Model file for the job. Use its own axes, mm. Face numbers are marked on the shaded views. A direction names the side the tool comes from. Give positions to 0.01 mm unless a question says otherwise; leave off trailing zeros. Loops run counter-clockwise (first coordinate to the right, second up) from the corner with the lowest first, then second, coordinate; pieces in that order, holes last. Notation, with made-up numbers: (-21, -2.5) - (29, -2.5) arc R29 cw to (29, 20.5) - close; hole circle Ø2 at (42, 1). An arc over 180 degrees is marked (long way). Use a Markdown table: item, result.
from build123d import *

# Parameters (mm, degrees)
EXTRUDE_1_DEPTH     = 60
SKETCH_3_W          = 10
SKETCH_3_H          = 40
CUT_EXTRUDE_2_DEPTH = 148.102218349
EXTRUDE_4_DEPTH     = 30
EXTRUDE_5_DEPTH     = 30
SKETCH_9_R          = 5
EXTRUDE_6_DEPTH     = 30
SKETCH_10_R         = 2.5
EXTRUDE_7_DEPTH     = 10
SKETCH_11_W         = 20.162650783
SKETCH_11_H         = 30
CUT_EXTRUDE_3_DEPTH = 10


with BuildPart() as part:
    # 草图1 → 凸台-拉伸1 (new body)
    with BuildSketch(Plane(origin=(0, 0, 0), x_dir=(1, 0, 0), z_dir=(0, 1, 0))):
        Polygon((0, 0), (120.162650783, 0), (120.162650783, 60), (100, 60), (100, 20), (0, 20), align=None)
    extrude(amount=EXTRUDE_1_DEPTH)

    # 草图3 → 切除-拉伸2 (cut, through all)
    with BuildSketch(Plane(origin=(120.162650783, 0, 0), x_dir=(0, 0, -1), z_dir=(1, 0, 0))):
        with Locations((55, 30)):
            Rectangle(SKETCH_3_W, SKETCH_3_H)
    extrude(amount=-CUT_EXTRUDE_2_DEPTH, mode=Mode.SUBTRACT)

    # 草图7 → 凸台-拉伸4 (add)
    with BuildSketch(Plane(origin=(0, 60, 0), x_dir=(1, 0, 0), z_dir=(0, 1, 0))):
        Polygon((0, 20), (0, 0), (120.162650783, 0), (120.162650783, 60), (100, 60), (100, 20), align=None)
    extrude(amount=EXTRUDE_4_DEPTH)

    # 草图8 → 凸台-拉伸5 (add)
    with BuildSketch(Plane.XZ):
        Polygon((0, -20), (0, 0), (120.162650783, 0), (120.162650783, -60), (100, -60), (100, -20), align=None)
    extrude(amount=EXTRUDE_5_DEPTH)

    # 草图9 → 凸台-拉伸6 (add)
    with BuildSketch(Plane(origin=(0, 0, -20), x_dir=(-1, 0, 0), z_dir=(0, 0, -1))):
        with Locations(Location((-10, -20, 0), (0, 0, 180))):
            Circle(SKETCH_9_R)
        with Locations(Location((-10, 80, 0), (0, 0, 180))):
            Circle(SKETCH_9_R)
    extrude(amount=EXTRUDE_6_DEPTH)

    # 草图10 → 凸台-拉伸7 (add)
    with BuildSketch(Plane(origin=(0, 0, -50), x_dir=(-1, 0, 0), z_dir=(0, 0, -1))):
        with Locations((-10, -20)):
            Circle(SKETCH_10_R)
        with Locations((-10, 80)):
            Circle(SKETCH_10_R)
    extrude(amount=EXTRUDE_7_DEPTH)

    # 草图11 → 切除-拉伸3 (cut)
    with BuildSketch(Plane(origin=(0, 0, -60), x_dir=(-1, 0, 0), z_dir=(0, 0, -1))):
        with Locations((-110.081325392, -5)):
            Rectangle(SKETCH_11_W, SKETCH_11_H)
        with Locations((-110.081325392, 65)):
            Rectangle(SKETCH_11_W, SKETCH_11_H)
    extrude(amount=-CUT_EXTRUDE_3_DEPTH, mode=Mode.SUBTRACT)


solid = part.part
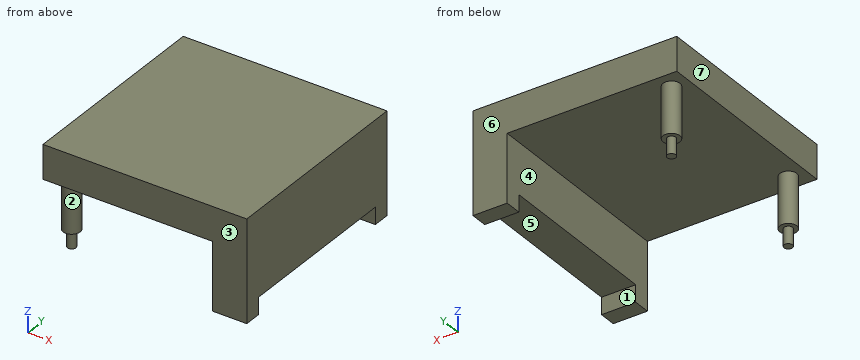
(1) Slice it at D-D, the plane x = 10. Write the cut outline in (y, z), plus the area to 3 significant figures.
Computed:
| item | result |
|---|---|
| outline | (-30, -20) - (-25, -20) - (-25, -50) - (-22.5, -50) - (-22.5, -60) - (-17.5, -60) - (-17.5, -50) - (-15, -50) - (-15, -20) - (75, -20) - (75, -50) - (77.5, -50) - (77.5, -60) - (82.5, -60) - (82.5, -50) - (85, -50) - (85, -20) - (90, -20) - (90, 0) - (-30, 0) - close |
| area | 3,100 mm² |
(2) Pin check, flat tips, straight feed: P1, Ø6, axis at x = 57, y = 3.5, coming from the -Z side; P2, Ø2, axis at y = 68.5, z = -40, coming from the -X side; P3, Ø6, axis at x = 113.5, y = 19, coming from the -Z side; P4, Ø1.5, axis at x = 102.5, y = -3.5, coming from the +Z side. Stop position of each tip, or through.
Computed:
| item | result |
|---|---|
| P1 | z = -20 |
| P2 | x = 100 |
| P3 | z = -50 |
| P4 | z = 0 |
(3) Drill centre lines: probe 1 along Z at (x, y) = (69.5, 65); probe 2 along X at (y, z) = (9, -34); probe 3 along Z at (x, y) = (101, 2.5). Where is each one in solid material? Low to high. Write a range as [from, to].
Computed:
| item | result |
|---|---|
| probe 1 | [-20, 0] |
| probe 2 | [100, 120.16] |
| probe 3 | [-50, 0] |
(4) 3-axis set-ups, long thin cutter, end or side, ignore diameter. For the marked faces 1, 2, 3 and 4: which of +Z, -Z, +X, -X, +Y, -Y reach the whole face in a straight line?
Computed:
| item | result |
|---|---|
| face 1 | -Z, +X |
| face 2 | -Z |
| face 3 | +Z, -Z, +X, -X, -Y |
| face 4 | -Z, +Y, -Y |
(5) Mould opens along Y. For the marked faces 5, 6 and 7 say: pulls with the +Y half, pulls with the -Y half, needs draft (parallel to the pull), parting line crosses it, or undercut.
Computed:
| item | result |
|---|---|
| face 5 | undercut |
| face 6 | pulls with the +Y half |
| face 7 | needs draft |
(6) Slice it at A-A, the plane z = -48.5. Write the cut outline in (x, y).
Computed:
| item | result |
|---|---|
| outline | circle Ø10 at (10, -20); circle Ø10 at (10, 80); (100, -30) - (120.16, -30) - (120.16, 90) - (100, 90) - close |
(7) Slice it at B-B, the plane x = 109.5. Write the cut outline in (y, z), plus the area to 3 significant figures.
Computed:
| item | result |
|---|---|
| outline | (-30, -60) - (-20, -60) - (-20, -50) - (80, -50) - (80, -60) - (90, -60) - (90, 0) - (-30, 0) - close |
| area | 6,200 mm² |
(8) Slice it at C-C, the plane y = 26. Write the cut outline in (x, z), plus the area to 3 significant figures.
Computed:
| item | result |
|---|---|
| outline | (0, -20) - (100, -20) - (100, -50) - (120.16, -50) - (120.16, 0) - (0, 0) - close |
| area | 3,010 mm² |
